Can you work these out from the model? Positions are in its coordinate system, mm. A direction names the side the tool comes from. Give positions to 0.01 mm unless a question says otherwise; leave off trailing zeros. Write each loop counter-clockwise with the first axis right and the second up, starting at its lowest first coordinate (ties: lowest second). Pieces come first, ordered by that corner, then holes.
1. Suppose I cut it at A-A (z = -20.5). Please give me the cut outline in (x, y).
2. Thinking about a two-plate mould opening in X: for faces 1 (the flat face through (-33, -4, -64)), 2 (the cylindrical face through (15.825, -2.465, -52.964)), 3 (the flat face through (-29, -6, -57)), which applies, pulls with the +X half, pulls with the -X half, needs draft (parallel to the pull), parting line crosses it, or undercut?
3. Suppose I cut it at B-B (x = 25). Please give me the cut outline in (y, z).
4. On a 3-axis mill with a long thin cutter (end or side, diameter ignored), from which of +Z, -Z, +X, -X, +Y, -Y can I reach the whole of each face in a straight line? I mean faces 4 (the flat face through (-29, -6, -15)), 5 (the flat face through (-21, -3, -36)), 6 (the flat face through (17, -6, -64)). Say none if no direction works.
5. Suppose I cut it at C-C (x = 0). Please give me the cut outline in (y, z), and give its area (3 significant figures).
6. I'm going to push flat-ended pins straight in: pin 1 (5 mm diameter, centred on y = -6.5, z = -30.5, fed in from +X); pin 2 (5 mm diameter, centred on x = -15.5, z = -51.5, fed in from -Y). Where does each tip first touch, or does it pass through?
7. Suppose I cut it at D-D (y = -9.75). Give the number of separate pieces and of enclosed holes in the cut face, and give its area (3 significant figures).
8. If I drill on probe 1 along Z at (x, y) = (15.5, -3.5); probe 2 along Z at (x, y) = (26.5, -15); probe 3 along Y at (x, z) = (25, -62), over which ranges is the centre line in solid material (lowest first)?
```python
from build123d import *

# Parameters (mm, degrees)
SKETCH1_R           = 4
BOSS_EXTRUDE1_DEPTH = 15
SKETCH2_W           = 42
SKETCH2_H           = 5
BOSS_EXTRUDE2_DEPTH = 42
BOSS_EXTRUDE3_START = -57
SKETCH1_2_R         = 4
BOSS_EXTRUDE3_DEPTH = 15
SKETCH3_R           = 1.5
SKETCH3_R_2         = 11
CUT_EXTRUDE1_DEPTH  = 81.802227692


with BuildPart() as part:
    # Sketch1 → Boss-Extrude1 (new body)
    with BuildSketch(Plane.XY):
        with BuildLine():
            Line((33, 0), (-33, 0))
            Line((-33, 0), (-33, -8))
            ThreePointArc((-33, -8), (-25, -16), (-17, -8))
            Line((-17, -8), (-17, -5))
            Line((-17, -5), (17, -5))
            Line((17, -5), (17, -8))
            ThreePointArc((17, -8), (25, -16), (33, -8))
            Line((33, -8), (33, 0))
        make_face()
        with Locations((-25, -8)):
            Circle(SKETCH1_R, mode=Mode.SUBTRACT)
        with Locations(Location((25, -8, 0), (0, 0, 180))):
            Circle(SKETCH1_R, mode=Mode.SUBTRACT)
    extrude(amount=-BOSS_EXTRUDE1_DEPTH)

    # Sketch2 → Boss-Extrude2 (add)
    with BuildSketch(Plane(origin=(0, 0, -15), x_dir=(-1, 0, 0), z_dir=(0, 0, -1))):
        with Locations((0, -2.5)):
            Rectangle(SKETCH2_W, SKETCH2_H)
    extrude(amount=BOSS_EXTRUDE2_DEPTH)

    # Sketch1<2> → Boss-Extrude3 (add)
    with BuildSketch(Plane.XY.offset(BOSS_EXTRUDE3_START)):
        with BuildLine():
            Line((33, 0), (-33, 0))
            Line((-33, 0), (-33, -8))
            ThreePointArc((-33, -8), (-25, -16), (-17, -8))
            Line((-17, -8), (-17, -5))
            Line((-17, -5), (17, -5))
            Line((17, -5), (17, -8))
            ThreePointArc((17, -8), (25, -16), (33, -8))
            Line((33, -8), (33, 0))
        make_face()
        with Locations((-25, -8)):
            Circle(SKETCH1_2_R, mode=Mode.SUBTRACT)
        with Locations(Location((25, -8, 0), (0, 0, 180))):
            Circle(SKETCH1_2_R, mode=Mode.SUBTRACT)
    extrude(amount=-BOSS_EXTRUDE3_DEPTH)

    # Sketch3 → Cut-Extrude1 (cut, through all)
    with BuildSketch(Plane(origin=(0, 0, 0), x_dir=(1, 0, 0), z_dir=(0, 1, 0))):
        with Locations(Location((-15.5, 51.5, 0), (0, 0, 180))):
            Circle(SKETCH3_R)
        with Locations(Location((0, 36, 0), (0, 0, 180))):
            Circle(SKETCH3_R_2)
        with Locations(Location((15.5, 51.5, 0), (0, 0, 180))):
            Circle(SKETCH3_R)
        with Locations(Location((15.5, 20.5, 0), (0, 0, 180))):
            Circle(SKETCH3_R)
        with Locations(Location((-15.5, 20.5, 0), (0, 0, 180))):
            Circle(SKETCH3_R)
    extrude(amount=-CUT_EXTRUDE1_DEPTH, mode=Mode.SUBTRACT)


solid = part.part
```
Checks:
1. outline: (-21, -5) - (-17, -5) - (-17, 0) - (-21, 0) - close; (-14, -5) - (14, -5) - (14, 0) - (-14, 0) - close; (17, -5) - (21, -5) - (21, 0) - (17, 0) - close
2. face 1: pulls with the -X half
2. face 2: undercut
2. face 3: needs draft
3. outline: (-16, -72) - (-12, -72) - (-12, -57) - (-16, -57) - close; (-16, -15) - (-12, -15) - (-12, 0) - (-16, 0) - close; (-4, -72) - (0, -72) - (0, -57) - (-4, -57) - close; (-4, -15) - (0, -15) - (0, 0) - (-4, 0) - close
4. face 4: -X, -Y
4. face 5: -X, +Y, -Y
4. face 6: +Z, -Z, -Y
5. outline: (-5, -72) - (0, -72) - (0, -47) - (-5, -47) - close; (-5, -25) - (0, -25) - (0, 0) - (-5, 0) - close
5. area: 250 mm2
6. pin 1: stops at x = 21
6. pin 2: stops at y = -5
7. separate pieces: 8
7. enclosed holes: 0
7. area: 505 mm2
8. probe 1: z = -72 to -53, -50 to -22, -19 to 0
8. probe 2: z = -72 to -57, -15 to 0
8. probe 3: y = -16 to -12, -4 to 0
